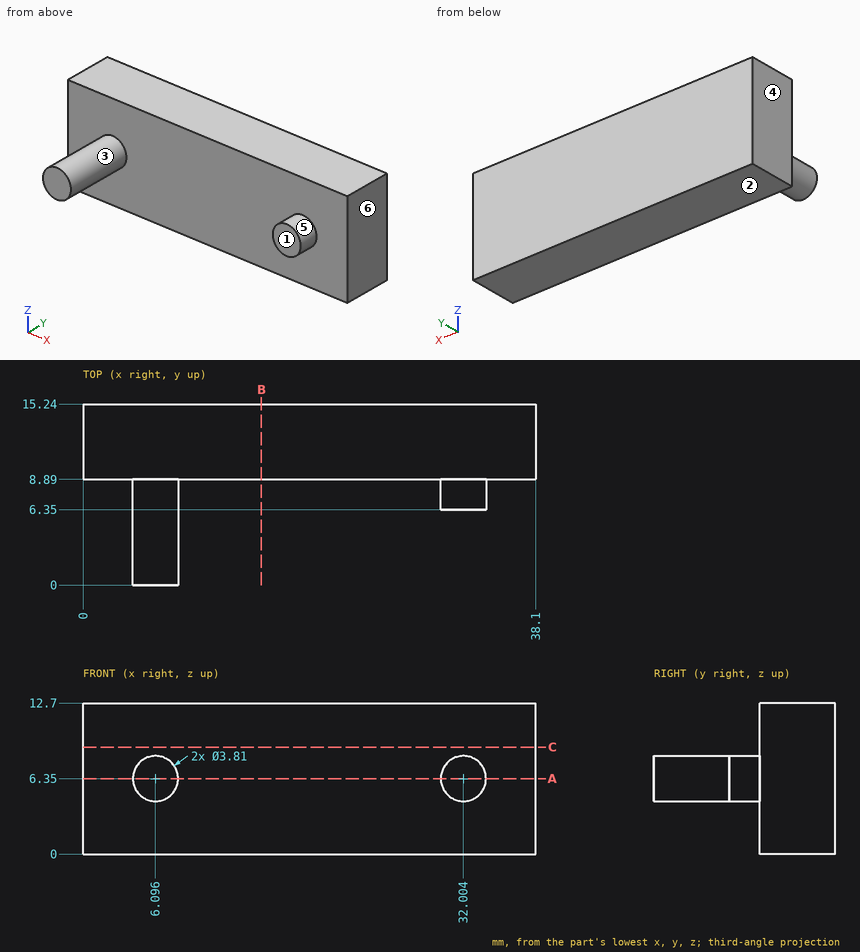
Part print with two shaded views. Sizes in mm from the minimum x, y, z corner. A direction names the side the tool comes from. Coordinates: 2 decimals unless noted, no trailing zeros. Order: outer loops, then holes, each group sorted by start corner. A loop starts at its lowest first (then second) coordinate and runs counter-clockwise, first axis right, second up. Notation, with made-up numbers: M 63,12.5 L 71,12.5 A17 ccw 71,36.5 Z; hole C 76,69.25 d6. An arc over 180 degrees is marked long. Use a Markdown table: item, result.
(1) Pull direction X, two halves, no side cores. Call the marked faces 4, 5 and 6: released by +X, released by -X, zero draft, split by the parting line, or undercut.
A:
| item | result |
|---|---|
| face 4 | released by -X |
| face 5 | undercut |
| face 6 | released by +X |
(2) Cut at B-B on x = 15. Write the cut outline in (y, z), then the cut area to 3 significant figures.
A:
| item | result |
|---|---|
| outline | M 8.89,0 L 15.24,0 L 15.24,12.7 L 8.89,12.7 Z |
| area | 80.6 mm^2 |
(3) Cut at A-A on z = 6.35. Write the cut outline in (x, y), then the cut area to 3 significant figures.
A:
| item | result |
|---|---|
| outline | M 0,8.89 L 4.19,8.89 L 4.19,0 L 8,0 L 8,8.89 L 30.1,8.89 L 30.1,6.35 L 33.91,6.35 L 33.91,8.89 L 38.1,8.89 L 38.1,15.24 L 0,15.24 Z |
| area | 285 mm^2 |
(4) Probe L1, parallel to Y at x = 28, z = 5.5; L2, parallel to X at y = 7, z = 6; L3, parallel to X at y = 8.75, z = 8. List the from-to ranges inside material, lowest first.
A:
| item | result |
|---|---|
| L1 | y = 8.89 to 15.24 |
| L2 | x = 4.22 to 7.97, 30.13 to 33.88 |
| L3 | x = 5.14 to 7.05, 31.05 to 32.96 |
(5) Cut at C-C on z = 9. Write the cut outline in (x, y).
A:
| item | result |
|---|---|
| outline | M 0,8.89 L 38.1,8.89 L 38.1,15.24 L 0,15.24 Z |
(6) Tool access for the marked faces 1, 2 and 3: list every direction of +Z, -Z, +X, -X, +Y, -Y with a clear straight run to the whole face (end or side of a thin tool).
A:
| item | result |
|---|---|
| face 1 | +Z, -Z, +X, -Y |
| face 2 | -Z, +X, -X, +Y, -Y |
| face 3 | -Y |
(7) Flat gauge pins, fed straight in: pin 1 (3 mm diameter, centred on x = 32.5, z = 6.5, fed in from -Y); pin 2 (2 mm diameter, centred on y = 2, z = 7, fed in from -X); pin 3 (1 mm diameter, centred on x = 29.5, z = 7, fed in from -Y). Where does each tip first touch, or does it go through?
A:
| item | result |
|---|---|
| pin 1 | stops at y = 6.35 |
| pin 2 | stops at x = 4.19 |
| pin 3 | stops at y = 8.89 |
